```python
from build123d import *

# Parameters (mm, degrees)
F2_R = 5


# Not quite as in the source:
# - a fillet or chamfer that OpenCascade refuses, or shapes differently, is made with other operations: its cross-section is extruded or revolved along the edge and cut away or added


with BuildPart() as f1:
    # F0 (on Front) → F1 (revolve)
    with BuildSketch(Plane.XZ):
        Polygon((-30.2233248949, 37.0877869427), (-36.4803494329, 36.5061946213), (-36.4803494329, -13.4938053787), (-34.2613953475, -13.4938053787), (-34.2613953475, -19.2220297002), (-36.4803494329, -19.2220297002), (-36.4803494329, -33.86637941), (-19.9121574584, -33.86637941), (0, -33.86637941), (0, -26.3013252845), (-30.2233248949, -26.3013252845), align=None)
    revolve(axis=Axis((0, 0, -30.0838523473), (0, 0, 1)))

    # F2
    f2_edges = [f1.edges().sort_by_distance(p)[0] for p in [
        (36.480349, 0, 36.506195),
    ]]
    fillet(f2_edges, radius=F2_R)

    # F3: fillet of radius 5 on 2 edges, made by hand

    # F3_s1 → F3_t2 (revolve, cut)
    with BuildSketch(Plane.XZ):
        with BuildLine():
            ThreePointArc((-31.9428428579, 36.9282346211), (-30.6731716306, 35.2277917828), (-30.2229248949, 33.1539430061))
            Line((-30.2229248949, 33.1539430061), (-29.7228023494, 33.1539430061))
            ThreePointArc((-29.7228023494, 33.1539430061), (-29.7232023494, 35.1208649744), (-29.7232023494, 37.0877869427))
            Line((-29.7232023494, 37.0877869427), (-30.2696119123, 37.5857629186))
            ThreePointArc((-30.2696119123, 37.5857629186), (-31.1293581124, 37.5058492495), (-31.6147121087, 37.3056637826))
            Line((-31.6147121087, 37.3056637826), (-31.9428428579, 36.9282346211))
        make_face()
    revolve(axis=Axis((0, 0, 37.0877869427), (0, 0, 1)), mode=Mode.SUBTRACT)


solid = f1.part
```
Verification items for the finished model (mm, model axes). A direction names the side the tool comes from. Give positions to 0.01 mm unless a question says otherwise; leave off trailing zeros. Loops run counter-clockwise (first coordinate to the right, second up) from the corner with the lowest first, then second, coordinate; pieces in that order, holes last. Notation, with made-up numbers: M 51.25,-8.75 L 85.25,-8.75 A27 cw 85.25,12.25 Z; hole C 67,54 d7. An arc over 180 degrees is marked long. One line per question, with ' | ' between items.
Item 1: Draft check along Z on faces 4 (the face through (0, 0, -26.301)), 5 (the face through (33, 11, -13.494)), 6 (the face through (-34.796, -10.958, -26.647)), 7 (the face through (-33, 11, -19.222)). Enter one of: +Z half, -Z half, draft (parallel to the pull), parting line (faces both ways), or undercut.
Completed:
face 4: +Z half | face 5: undercut | face 6: draft | face 7: undercut
Item 2: Section check A-A, the plane z = 7. Record the cut outline in (x, y), plus the area to 3 significant figures.
Completed:
outline: C 0,0 d72.96; hole C 0,0 d60.45 | area: 1,310 mm^2
Item 3: Thickness scan on line 1 (Y direction, x = 0, z = -2.5); line 2 (Z direction, x = -26, y = 15). Record the ranges inside material, lowest first. Write a range as [from, to].
Completed:
line 1: y = [-36.48, -30.22], [30.22, 36.48] | line 2: z = [-33.87, -26.3]
Item 4: Tool access check on faces 1 (the face through (-32.68, -10.29, -16.4)), 2 (the face through (-27.919, 11.576, 3.875)), 3 (the face through (1, -1, -33.866)). Record the directions out of +Z, -Z, +X, -X, +Y, -Y that give a thin tool (end or side, any length) a straight path to the whole face; none if there is none.
Completed:
face 1: none | face 2: +Z | face 3: -Z, +X, -X, +Y, -Y
Item 5: Depth check by flat-ended pin: P1, Ø5, axis at x = -6.5, z = 2.5, coming from the +Y side; P2, Ø8, axis at x = -5, z = -23, coming from the -Y side; P3, Ø8, axis at y = -7.5, z = -15.5, coming from the +X side. Enter the tip coordinate at first touch or a pass-through.
Completed:
P1: stops at y = 36.26 | P2: stops at y = -36.47 | P3: stops at x = 36.26
